The drawing under review shows one solid part. Ordinate dimensions are in mm from its lowest x, y, z. A direction names the side the tool comes from. Give positions to 0.01 mm unless a question says otherwise; leave off trailing zeros. Loops run counter-clockwise (first coordinate to the right, second up) from the corner with the lowest first, then second, coordinate; pieces in that order, holes last. Notation, with made-up numbers: M 44,-38.75 L 101,-38.75 A20 cw 101,-23.75 Z; hole C 38.5,19 d7. An arc over 180 degrees is marked long. Write item = value, one per line. Start each with the question number.
1. We need section C-C on x = 13.5. Give the boundary of the cut face in (y, z).
2. For pin 1 (3 mm diameter, centred on x = 15, z = 11, fed in from -Y); pin 2 (5 mm diameter, centred on x = 23, z = 10.5, fed in from -Y), all flat-tipped, find the tip position at first contact; note any pin that passes through.
3. We need section A-A on z = 8.25. Give the boundary of the cut face in (x, y).
4. Wall thickness on line 1 along Z through (x, y) = (24.25, 12); line 2 along Y through (x, z) = (16.5, 9.25); line 3 along Y through (x, z) = (5, 9.25): over which ranges is each line inside the solid? List them lowest first. Write a range as from..to.
5. We need section B-B on y = 21. Give the boundary of the cut face in (x, z), then the cut area to 3 significant figures.
6. For the marked faces 1, 2 and 3, list the 3-axis set-ups (+Z, -Z, +X, -X, +Y, -Y) from which the entire face can be reached by the end or side of a thin tool; tool diameter is ignored.
7. We need section D-D on x = 4. Give the boundary of the cut face in (y, z), then the cut area to 3 significant figures.
8. Draft analysis for pull direction X (two halves, no side actions). For the marked faces 4, 5, 6 and 7, state which applies: pulls with the +X half, pulls with the -X half, needs draft (parallel to the pull), parting line crosses it, or undercut.
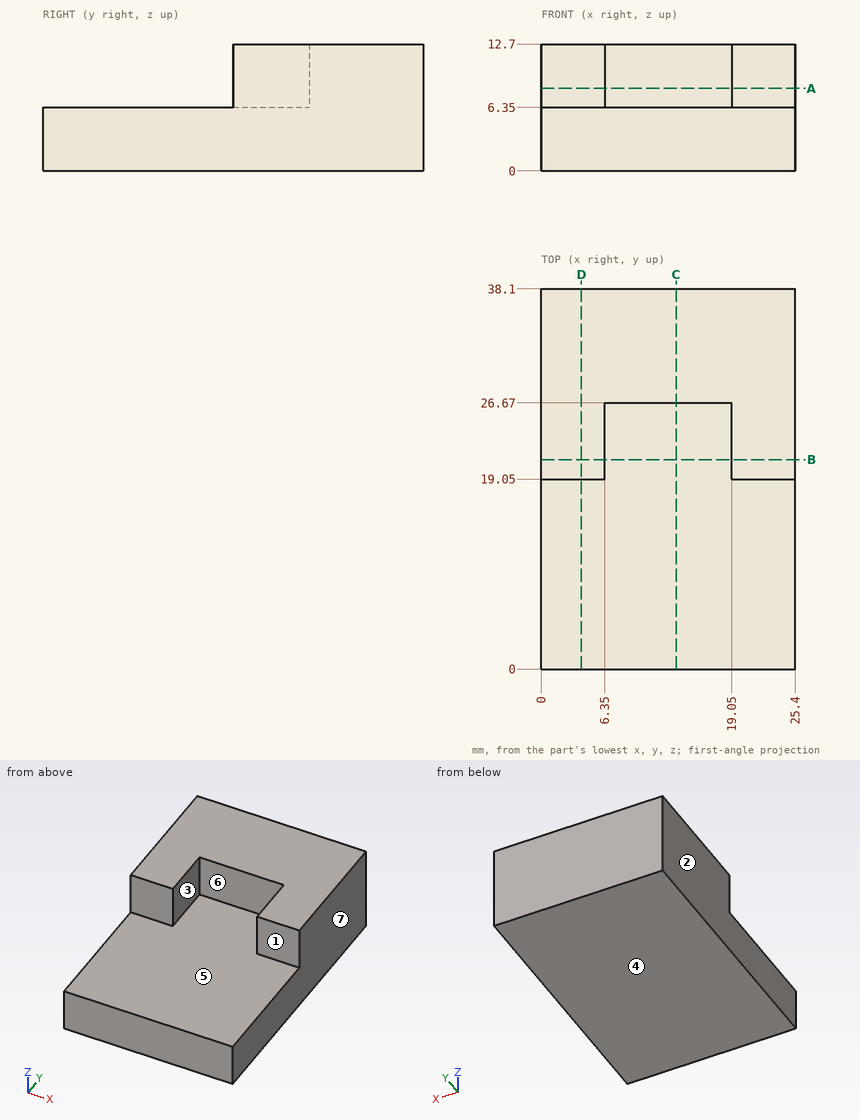
Final values:
q1.outline = M 0,0 L 38.1,0 L 38.1,12.7 L 26.67,12.7 L 26.67,6.35 L 0,6.35 Z
q2.pin_1 = 26.67
q2.pin_2 = 19.05
q3.outline = M 0,19.05 L 6.35,19.05 L 6.35,26.67 L 19.05,26.67 L 19.05,19.05 L 25.4,19.05 L 25.4,38.1 L 0,38.1 Z
q4.line_1 = 0..6.35
q4.line_2 = 26.67..38.1
q4.line_3 = 19.05..38.1
q5.outline = M 0,0 L 25.4,0 L 25.4,12.7 L 19.05,12.7 L 19.05,6.35 L 6.35,6.35 L 6.35,12.7 L 0,12.7 Z
q5.area = 242 mm²
q6.face_1 = +Z, +X, -X, -Y
q6.face_2 = +Z, -Z, -X, +Y, -Y
q6.face_3 = +Z, -Y
q7.outline = M 0,0 L 38.1,0 L 38.1,12.7 L 19.05,12.7 L 19.05,6.35 L 0,6.35 Z
q7.area = 363 mm²
q8.face_4 = needs draft
q8.face_5 = undercut
q8.face_6 = undercut
q8.face_7 = pulls with the +X half
